```python
from build123d import *

# Parameters (mm, degrees)
SKETCH1_R                      = 17.5
BOSS_EXTRUDE1_DEPTH            = 2.5
CUT_EXTRUDE1_DEPTH             = 25.874685928
FILLET2_R                      = 0.3
CIRPATTERN1_COUNT              = 20
THROUGH_CENTER_HOLE_DEPTH      = 25.802421489
THROUGH_CENTER_HOLE_DEPTH_BACK = 25.802421489
SKETCH4_R                      = 1.25
TO_KNUCKLE_MOUNT_DEPTH         = 25.802421489
TO_KNUCKLE_MOUNT_DEPTH_BACK    = 25.802421489
SKETCH5_R                      = 1.65


with BuildPart() as part:
    # Sketch1 → Boss-Extrude1 (new, symmetric)
    with BuildSketch(Plane.XY):
        Circle(SKETCH1_R)
    extrude(amount=BOSS_EXTRUDE1_DEPTH, both=True)

    # Sketch3 → Cut-Extrude1 (cut, symmetric)
    with BuildSketch(Plane.XY):
        with BuildLine():
            ThreePointArc((-2.489947944, 18.331670934), (-1.138475024, 17.178633755), (-0.590517817, 15.488747164))
            ThreePointArc((-0.590517817, 15.488747164), (0, 15.5), (0.590517817, 15.488747164))
            ThreePointArc((0.590517817, 15.488747164), (1.138475024, 17.178633755), (2.489947944, 18.331670934))
            ThreePointArc((2.489947944, 18.331670934), (0, 18.5), (-2.489947944, 18.331670934))
        make_face()
    cut_extrude1 = extrude(amount=CUT_EXTRUDE1_DEPTH, both=True, mode=Mode.SUBTRACT)

    # Fillet2
    fillet2_edges = [part.edges().sort_by_distance(p)[0] for p in [
        (-0.590517817, 15.488747164, 0),
        (0.590517817, 15.488747164, 0),
    ]]
    fillet(fillet2_edges, radius=FILLET2_R)

    # CirPattern1: Cut-Extrude1 ×20 about axis
    cirpattern1_axis = Axis((0, 0, 0), (0, 0, 1))
    for i in range(1, CIRPATTERN1_COUNT):
        add(cut_extrude1.rotate(cirpattern1_axis, i * 360 / CIRPATTERN1_COUNT), mode=Mode.SUBTRACT)

    # Sketch4 → Through_Center_Hole (cut, two sides: drawn at the far end of the back side and taken through both)
    with BuildSketch(Plane.XY.offset(-THROUGH_CENTER_HOLE_DEPTH_BACK)):
        Circle(SKETCH4_R)
    extrude(amount=THROUGH_CENTER_HOLE_DEPTH + THROUGH_CENTER_HOLE_DEPTH_BACK, mode=Mode.SUBTRACT)

    # Sketch5 → To_Knuckle_Mount (cut, two sides: drawn at the far end of the back side and taken through both)
    with BuildSketch(Plane.XY.offset(-TO_KNUCKLE_MOUNT_DEPTH_BACK)):
        with Locations((9, 0)):
            Circle(SKETCH5_R)
        with Locations((-9, 0)):
            Circle(SKETCH5_R)
    extrude(amount=TO_KNUCKLE_MOUNT_DEPTH + TO_KNUCKLE_MOUNT_DEPTH_BACK, mode=Mode.SUBTRACT)


solid = part.part
```
Source: CAD feature listing. Evaluate the final solid. Frame: model axes, mm. A direction names the side the tool comes from. Round coordinates to 2 decimals unless told otherwise and drop trailing zeros. Loops run counter-clockwise (first coordinate to the right, second up) from the corner with the lowest first, then second, coordinate; pieces in that order, holes last. Notation, with made-up numbers: M 22,74.5 L 47,74.5 A12 ccw 47,92.5 Z; hole C 76.5,30.5 d8. An arc over 180 degrees is marked long. Use a Markdown table: item, result. Add a question column.
1. Mould query, pull axis X, two halves, no side actions, for faces 1 (the cylindrical face through (4.343, 15.985, 0.035)), 2 (the cylindrical face through (12.36, -12.39, 0.04)), 3 (the cylindrical face through (-16.544, -0.809, 0.035)). Classes: pulls with the +X half, pulls with the -X half, needs draft (parallel to the pull), parting line crosses it, or undercut.
2. Reachability of faces 4 (the cylindrical face through (-15.46, 5.86, 0.04)), 5 (the cylindrical face through (16.52, -0.8, 0.04)), 6 (the cylindrical face through (12.545, -9.104, 0.035)), 7 (the cylindrical face through (0.809, -16.544, 0.035)) from +Z, -Z, +X, -X, +Y, -Y: full face, straight path, thin tool, end or side. Return the list, or none.
3. Section query C-C on y = 10. Return the cut outline in (x, z).
4. Section query A-A on y = 0. Return the cut outline in (x, z), then the cut area to 4 significant figures.
5. Line query: line 1 (X direction, y = 0, z = -0.8); line 2 (Y direction, x = 0, z = 2.2); line 3 (X direction, y = -12.5, z = -1.75). Output: solid intervals per line, ascending.
6. Section query B-B on z = -1.3. Give the number of separate pieces and of enclosed holes in the cut face, then the cut area to 3 significant figures.
7. Contact query for flat-ended pins moving along their axis: P1, Ø3, axis at x = 11, z = -2, coming from the -Y side; P2, Ø1.5, axis at x = 3, z = 0.5, coming from the +Y side. Output: stop coordinate, or through.
Reported:
| question | item | result |
|---|---|---|
| 1 | face 1 | undercut |
| 1 | face 2 | pulls with the +X half |
| 1 | face 3 | pulls with the -X half |
| 2 | face 4 | +Z, -Z, -X |
| 2 | face 5 | +Z, -Z, +X |
| 2 | face 6 | +Z, -Z |
| 2 | face 7 | +Z, -Z, -Y |
| 3 | outline | M -12.62,-2.5 L 12.62,-2.5 L 12.62,2.5 L -12.62,2.5 Z |
| 4 | outline | M -15.5,-2.5 L -10.65,-2.5 L -10.65,2.5 L -15.5,2.5 Z; M -7.35,-2.5 L -1.25,-2.5 L -1.25,2.5 L -7.35,2.5 Z; M 1.25,-2.5 L 7.35,-2.5 L 7.35,2.5 L 1.25,2.5 Z; M 10.65,-2.5 L 15.5,-2.5 L 15.5,2.5 L 10.65,2.5 Z |
| 4 | area | 109.5 mm² |
| 5 | line 1 | x = -15.5 to -10.65, -7.35 to -1.25, 1.25 to 7.35, 10.65 to 15.5 |
| 5 | line 2 | y = -15.5 to -1.25, 1.25 to 15.5 |
| 5 | line 3 | x = -12.25 to -9.87, -9.17 to 9.17, 9.87 to 12.25 |
| 6 | separate pieces | 1 |
| 6 | enclosed holes | 3 |
| 6 | area | 873 mm² |
| 7 | P1 | stops at y = -13.33 |
| 7 | P2 | stops at y = 17.35 |
